For this review, take the finished solid that the model builds, in its own axes (mm). Coordinates: 2 decimals unless noted, no trailing zeros. Loops run counter-clockwise (first coordinate to the right, second up) from the corner with the lowest first, then second, coordinate; pieces in that order, holes last. Notation, with made-up numbers: (53, 47) - (91, 47) arc R19 cw to (91, 69) - close; hole circle Ø4 at (41.25, -9.75). An arc over 180 degrees is marked (long way). Answer as a JSON object with one key per item and string values. Group by question number.
Item 1: To check wall thickness, follow line 1 (X direction, y = 14, z = 1.5); line 2 (Y direction, x = 5, z = 0.7); line 3 (Y direction, x = 17.5, z = 0.7) (3 decimals). State the ranges of each line that lie inside material, in increasing order.
Item 2: We need section B-B (y = 17). Give the boundary of the cut face in (x, z), then the cut area to 3 significant figures.
Item 3: We need section D-D (x = 20). Give the boundary of the cut face in (y, z).
Item 4: We need section C-C (x = 70). Give the boundary of the cut face in (y, z).
Item 5: We need section A-A (x = 46.5). Give the boundary of the cut face in (y, z).
from build123d import *

# Parameters (mm, degrees)
SKETCH_1_W          = 75
SKETCH_1_H          = 33.7
SKETCH_1_R          = 1.45
SKETCH_1_R_2        = 2
EXTRUDE_1_DEPTH     = 3
SKETCH_2_W          = 25.5
SKETCH_2_H          = 21.7
SKETCH_2_W_2        = 10.5
CUT_EXTRUDE_1_DEPTH = 10
FILLET_1_R          = 2.5
FILLET_2_R          = 3


with BuildPart() as part:
    # 草图1 → 凸台-拉伸1 (new body)
    with BuildSketch(Plane.XY):
        with Locations((37.5, 16.85)):
            Rectangle(SKETCH_1_W, SKETCH_1_H)
        with Locations((5, 17)):
            Circle(SKETCH_1_R, mode=Mode.SUBTRACT)
        with Locations((5, 5)):
            Circle(SKETCH_1_R, mode=Mode.SUBTRACT)
        with Locations((70, 17)):
            Circle(SKETCH_1_R, mode=Mode.SUBTRACT)
        with Locations((70, 5)):
            Circle(SKETCH_1_R, mode=Mode.SUBTRACT)
        with Locations((20, 17)):
            Circle(SKETCH_1_R_2, mode=Mode.SUBTRACT)
    extrude(amount=EXTRUDE_1_DEPTH)

    # 草图2 → 切除-拉伸1 (cut)
    with BuildSketch(Plane.XY.offset(3)):
        Polygon((4, 28.7), (20, 28.7), (14, 17.7), align=None)
        with Locations((53.25, 16.85)):
            Rectangle(SKETCH_2_W, SKETCH_2_H)
        with Locations((29.25, 16.85)):
            Rectangle(SKETCH_2_W_2, SKETCH_2_H)
        Polygon((5, 11.666666667), (16, 14), (20, 5), (10, 5), align=None)
    extrude(amount=-CUT_EXTRUDE_1_DEPTH, mode=Mode.SUBTRACT)

    # 圆角1
    fillet_1_edges = [part.edges().sort_by_distance(p)[0] for p in [
        (40.5, 6, 1.5),
        (40.5, 27.7, 1.5),
        (66, 27.7, 1.5),
        (66, 6, 1.5),
        (10, 5, 1.5),
        (5, 11.666666667, 1.5),
        (16, 14, 1.5),
        (20, 5, 1.5),
        (14, 17.7, 1.5),
        (4, 28.7, 1.5),
        (20, 28.7, 1.5),
        (24, 6, 1.5),
        (24, 27.7, 1.5),
        (34.5, 27.7, 1.5),
        (34.5, 6, 1.5),
    ]]
    fillet(fillet_1_edges, radius=FILLET_1_R)

    # 圆角2
    fillet_2_edges = [part.edges().sort_by_distance(p)[0] for p in [
        (0, 33.7, 1.5),
        (75, 33.7, 1.5),
        (75, 0, 1.5),
        (0, 0, 1.5),
    ]]
    fillet(fillet_2_edges, radius=FILLET_2_R)


solid = part.part
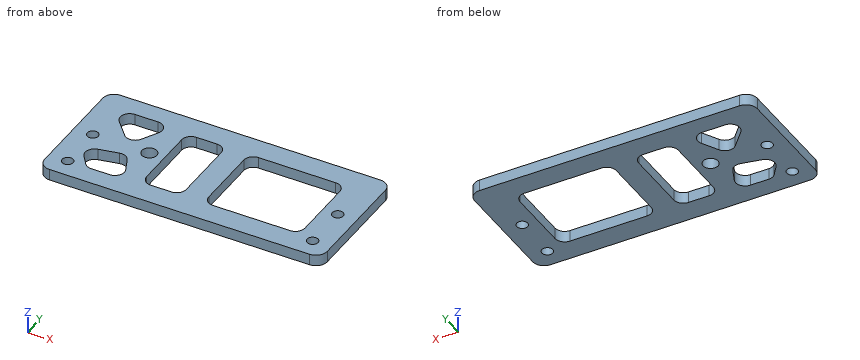
Check sheet entries:
{
 "1": {"line 1": "x = 0 to 24, 34.5 to 40.5, 66 to 75", "line 2": "y = 0 to 3.55, 6.45 to 15.55, 18.45 to 33.7", "line 3": "y = 0 to 5.394, 10.625 to 24.117, 28.022 to 33.7"},
 "2": {"outline": "(0, 0) - (3.55, 0) - (3.55, 3) - (0, 3) - close; (6.45, 0) - (18, 0) - (18, 3) - (6.45, 3) - close; (22, 0) - (24, 0) - (24, 3) - (22, 3) - close; (34.5, 0) - (40.5, 0) - (40.5, 3) - (34.5, 3) - close; (66, 0) - (68.55, 0) - (68.55, 3) - (66, 3) - close; (71.45, 0) - (75, 0) - (75, 3) - (71.45, 3) - close", "area": "87.6 mm2"},
 "3": {"outline": "(0, 0) - (15, 0) - (15, 3) - (0, 3) - close; (19, 0) - (33.7, 0) - (33.7, 3) - (19, 3) - close"},
 "4": {"outline": "(0, 0) - (3.55, 0) - (3.55, 3) - (0, 3) - close; (6.45, 0) - (15.55, 0) - (15.55, 3) - (6.45, 3) - close; (18.45, 0) - (33.7, 0) - (33.7, 3) - (18.45, 3) - close"},
 "5": {"outline": "(0, 0) - (6, 0) - (6, 3) - (0, 3) - close; (27.7, 0) - (33.7, 0) - (33.7, 3) - (27.7, 3) - close"}
}
